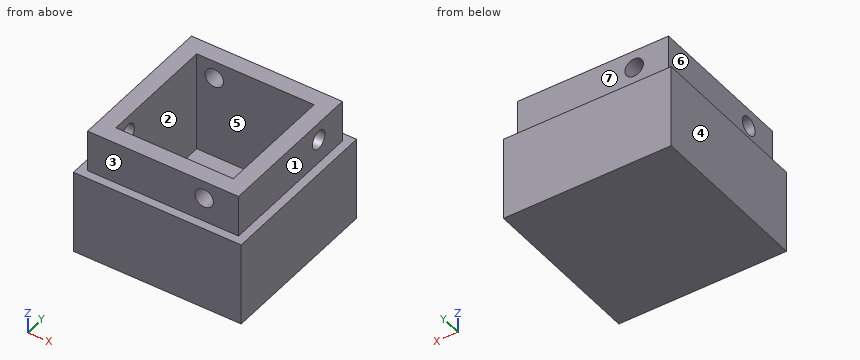
```python
from build123d import *

# Parameters (mm, degrees)
F2_W      = 20
F2_H      = 20
F3_DEPTH  = 3
F4_W      = 20
F4_H      = 20
F4_W_2    = 14
F4_H_2    = 14
F5_DEPTH  = 7
F7_W      = 18
F7_H      = 18
F7_W_2    = 14
F7_H_2    = 14
F8_DEPTH  = 5
F9_R      = 1.1
F10_DEPTH = 2
F11_R     = 1.1
F12_DEPTH = 3
F13_R     = 1.1
F14_DEPTH = 3
F15_R     = 1.1
F16_DEPTH = 3


with BuildPart() as f3:
    # F2 (on Top) → F3 (new body)
    with BuildSketch(Plane.XY):
        with Locations((10, -10)):
            Rectangle(F2_W, F2_H)
    extrude(amount=F3_DEPTH)

    # F4 (on face) → F5 (join)
    with BuildSketch(Plane.XY.offset(3)):
        with Locations((10, -10)):
            Rectangle(F4_W, F4_H)
        with Locations((10, -10)):
            Rectangle(F4_W_2, F4_H_2, mode=Mode.SUBTRACT)
    extrude(amount=F5_DEPTH)

    # F7 (on face) → F8 (join)
    with BuildSketch(Plane.XY.offset(10)):
        with Locations((10, -10)):
            Rectangle(F7_W, F7_H)
        with Locations((10, -10)):
            Rectangle(F7_W_2, F7_H_2, mode=Mode.SUBTRACT)
    extrude(amount=F8_DEPTH)

    # F9 (on face) → F10 (cut)
    with BuildSketch(Plane(origin=(0, -17, 0), x_dir=(-1, 0, 0), z_dir=(0, 1, 0))):
        with Locations((-14.9, 12.9)):
            Circle(F9_R)
    extrude(amount=-F10_DEPTH, mode=Mode.SUBTRACT)

    # F11 (on face) → F12 (cut)
    with BuildSketch(Plane.YZ.offset(3)):
        with Locations((-14.9, 12.9)):
            Circle(F11_R)
    extrude(amount=-F12_DEPTH, mode=Mode.SUBTRACT)

    # F13 (on face) → F14 (cut)
    with BuildSketch(Plane.XZ.offset(3)):
        with Locations((5.1, 12.9)):
            Circle(F13_R)
    extrude(amount=-F14_DEPTH, mode=Mode.SUBTRACT)

    # F15 (on face) → F16 (cut)
    with BuildSketch(Plane(origin=(17, 0, 0), x_dir=(0, -1, 0), z_dir=(-1, 0, 0))):
        with Locations((5.1, 12.9)):
            Circle(F15_R)
    extrude(amount=-F16_DEPTH, mode=Mode.SUBTRACT)


solid = f3.part
```
Can you work these out from the model? Positions are in its coordinate system, mm. Face numbers are marked on the shaded views. A direction names the side the tool comes from. Give positions to 0.01 mm unless a question says otherwise; leave off trailing zeros. Loops run counter-clockwise (first coordinate to the right, second up) from the corner with the lowest first, then second, coordinate; pieces in that order, holes last. Notation, with made-up numbers: M -8,-29 L 0,-29 A24 ccw 0,5 Z; hole C 1.25,30.5 d3. An arc over 180 degrees is marked long. One line per item, written item: value.
(1) We'd pull the mould along Y, two halves only. Please class the marked faces 5, 6 and 7: released by +Y, released by -Y, zero draft, split by the parting line, or undercut.
Returned:
face 5: undercut
face 6: zero draft
face 7: released by +Y
(2) Which directions (+Z, -Z, +X, -X, +Y, -Y) give clear straight access to the entire face, cutting with the end or side of a thin tool? Please do the marked faces 1, 2, 3 and 4.
Returned:
face 1: +Z, +X, +Y, -Y
face 2: +Z
face 3: +Z, +X, -X, -Y
face 4: +Z, -Z, -X, +Y, -Y
(3) I need wall thicknesses on line 1 (Y direction, x = 5.5, z = 3.5); line 2 (Z direction, x = 5.1, y = -2.1); line 3 (Y direction, x = 8, z = 12.5). Which ranges of each line are inside material? Lowest first, please.
Returned:
line 1: -20 to -17, -3 to 0
line 2: 0 to 11.8, 14 to 15
line 3: -19 to -17, -3 to -1
(4) Suppose I cut it at C-C on x = 14.9. List the corners of the cut face in (y, z) for me, plus the area to 3 significant figures.
Returned:
outline: M -20,0 L 0,0 L 0,10 L -1,10 L -1,15 L -3,15 L -3,3 L -17,3 L -17,11.8 L -19,11.8 L -19,10 L -20,10 Z; M -19,14 L -17,14 L -17,15 L -19,15 Z
area: 118 mm^2
(5) Will these pins go through, and if not, where does the flat tip stop? pin 1 (4 mm diameter, centred on x = 8.5, y = -10.5, fed in from +Z); pin 2 (3 mm diameter, centred on y = -14.9, z = 12.9, fed in from -X); pin 3 (2.5 mm diameter, centred on y = -10, z = 13, fed in from +X).
Returned:
pin 1: z = 3
pin 2: x = 1
pin 3: x = 19
(6) Suppose I cut it at D-D on y = -2.25. List the corners of the cut face in (x, z) for me, plus the area to 3 significant figures.
Returned:
outline: M 0,0 L 20,0 L 20,10 L 19,10 L 19,15 L 1,15 L 1,10 L 0,10 Z; hole C 5.1,12.9 d2.2
area: 286 mm^2
(7) Suppose I cut it at A-A on y = -14.9. List the corners of the cut face in (x, z) for me.
Returned:
outline: M 0,0 L 20,0 L 20,10 L 19,10 L 19,15 L 17,15 L 17,3 L 3,3 L 3,11.8 L 1,11.8 L 1,10 L 0,10 Z; M 1,14 L 3,14 L 3,15 L 1,15 Z
(8) Suppose I cut it at B-B on z = 12.9. List the corners of the cut face in (x, y) for me, plus the area to 3 significant figures.
Returned:
outline: M 1,-19 L 13.8,-19 L 13.8,-17 L 3,-17 L 3,-16 L 1,-16 Z; M 1,-13.8 L 3,-13.8 L 3,-3 L 4,-3 L 4,-1 L 1,-1 Z; M 6.2,-3 L 17,-3 L 17,-4 L 19,-4 L 19,-1 L 6.2,-1 Z; M 16,-19 L 19,-19 L 19,-6.2 L 17,-6.2 L 17,-17 L 16,-17 Z
area: 110 mm^2
